The listing builds one solid part. Answer for the finished solid, in the listing's coordinates (mm). Face numbers are marked on the shaded views. A direction names the side the tool comes from. Round coordinates to 2 decimals unless told otherwise and drop trailing zeros. Order: outer loops, then holes, each group sorted by start corner. A loop starts at its lowest first (then second) coordinate and runs counter-clockwise, first axis right, second up. Notation, with made-up numbers: M -6.75,28 L 42.25,28 A32 ccw 42.25,58 Z; hole C 86.5,18 d8. An arc over 180 degrees is marked long. Put each result on its own line as item: value. Start each with the question number.
1. Each of these flat-tipped pins is pushed along its axis until it touches: pin 1 Ø8 at (y, z) = (-6.5, 25.5) entering from +X; pin 2 Ø1.5 at (x, z) = (20.5, 53.5) entering from -Y; pin 3 Ø6.5 at (x, y) = (-15, 10.5) entering from -Z; pin 4 Ø3 at (x, z) = (-17.5, -45) entering from -Y. Where does it stop, or does it pass through?
2. Which of the six approach directions +Z, -Z, +X, -X, +Y, -Y give full straight-line access (tool end or side, diameter ignored) to the marked faces 4, 5 and 6?
3. The mould has two halves that part along Z. Classify the marked faces 1, 2 and 3: +Z half, -Z half, draft (parallel to the pull), parting line (faces both ways), or undercut.
4. The part is cut by section B-B (x = 10). Give the vertices of the cut face in (y, z), then the cut area to 3 significant figures.
5. Consider line 1 (X direction, y = 1.5, z = -45); line 2 (X direction, y = 5.5, z = 9); line 3 (X direction, y = 10, z = 57). Determine where each line is inside the solid, lowest interval first.
6. The part is cut by section C-C (z = 32). Give the vertices of the cut face in (x, y).
7. The part is cut by section D-D (y = 10.5). Give the vertices of the cut face in (x, z), then the cut area to 3 significant figures.
8. The part is cut by section A-A (y = -3). Give the vertices of the cut face in (x, z), then the cut area to 3 significant figures.
from build123d import *

# Parameters (mm, degrees)
ESBO_O1_W                 = 90
ESBO_O1_H                 = 100
RESSALTO_EXTRUS_O1_DEPTH  = 3
ESBO_O4_W                 = 20
ESBO_O4_H                 = 20
CORTE_EXTRUS_O1_DEPTH     = 3
DOBRA_START               = -30
DOBRA_ESBO_ADA1_DEPTH     = 80
DOBRA_ESBO_ADA1_2_DEPTH   = 80
DOBRA_ESBO_ADA2_DEPTH     = 80
DOBRA_ESBO_ADA2_2_DEPTH   = 80
FILETE1_R                 = 5
CHANFRO1_SIZE             = 5
FILETE2_R                 = 2.5
ESBO_O7_R                 = 2.5
CORTE_EXTRUS_O2_DEPTH     = 3
RESSALTO_EXTRUS_O2_DEPTH  = 21.5
ESBO_O9_W                 = 37
ESBO_O9_H                 = 15
CORTE_EXTRUS_O7_DEPTH     = 90
ESBO_O10_W                = 3
ESBO_O10_H                = 20
RESSALTO_EXTRUS_O3_DEPTH  = 30
FURO_ROSCADO_DE_M51_D     = 4.2
FURO_ROSCADO_DE_M51_DEPTH = 14
FURO_ROSCADO_DE_M51_TIP   = 1.2618073


# Read off the part's stored shape, not the designer's step: Dobra esboçada1, Dobra esboçada2
with BuildPart() as part:
    # Esboço1 → Ressalto-extrusão1 (new body)
    with BuildSketch(Plane(origin=(0, 0, 0), x_dir=(1, 0, 0), z_dir=(0, 1, 0))):
        Rectangle(ESBO_O1_W, ESBO_O1_H)
    extrude(amount=RESSALTO_EXTRUS_O1_DEPTH)

    # Esboço4 → Corte-extrusão1 (cut)
    with BuildSketch(Plane(origin=(0, 3, 0), x_dir=(1, 0, 0), z_dir=(0, 1, 0))):
        with Locations((-35, 40)):
            Rectangle(ESBO_O4_W, ESBO_O4_H)
        with Locations((35, 40)):
            Rectangle(ESBO_O4_W, ESBO_O4_H)
    extrude(amount=-CORTE_EXTRUS_O1_DEPTH, mode=Mode.SUBTRACT)

    # Dobra esboçada1 outline → Dobra esboçada1 (cut)
    with BuildSketch(Plane.XY.offset(DOBRA_START)):
        with BuildLine():
            Line((-45, 0), (-28.872983346, 0))
            ThreePointArc((-28.872983346, 0), (-27.449489743, 2.16227766), (-25, 3))
            Line((-25, 3), (-45, 3))
            Line((-45, 3), (-45, 0))
        make_face()
    extrude(amount=DOBRA_ESBO_ADA1_DEPTH, mode=Mode.SUBTRACT)

    # Dobra esbo_ada1 2 outline → Dobra esbo_ada1 2 (add)
    with BuildSketch(Plane.XY.offset(DOBRA_START)):
        with BuildLine():
            ThreePointArc((-28.872983346, 0), (-28.968118785, -0.49598283), (-29, -1))
            Line((-29, -1), (-29, -17.073009183))
            Line((-29, -17.073009183), (-26, -17.073009183))
            Line((-26, -17.073009183), (-26, -1))
            ThreePointArc((-26, -1), (-25.707106781, -0.292893219), (-25, 0))
            Line((-25, 0), (-28.872983346, 0))
        make_face()
    extrude(amount=DOBRA_ESBO_ADA1_2_DEPTH)

    # Dobra esboçada2 outline → Dobra esboçada2 (cut)
    with BuildSketch(Plane.XY.offset(DOBRA_START)):
        with BuildLine():
            ThreePointArc((25, 3), (27.449489743, 2.16227766), (28.872983346, 0))
            Line((28.872983346, 0), (45, 0))
            Line((45, 0), (45, 3))
            Line((45, 3), (25, 3))
        make_face()
    extrude(amount=DOBRA_ESBO_ADA2_DEPTH, mode=Mode.SUBTRACT)

    # Dobra esbo_ada2 2 outline → Dobra esbo_ada2 2 (add)
    with BuildSketch(Plane.XY.offset(DOBRA_START)):
        with BuildLine():
            Line((26, -1), (26, -17.073009183))
            Line((26, -17.073009183), (29, -17.073009183))
            Line((29, -17.073009183), (29, -1))
            ThreePointArc((29, -1), (28.968118785, -0.49598283), (28.872983346, 0))
            Line((28.872983346, 0), (25, 0))
            ThreePointArc((25, 0), (25.707106781, -0.292893219), (26, -1))
        make_face()
    extrude(amount=DOBRA_ESBO_ADA2_2_DEPTH)

    # Filete1
    filete1_edges = [part.edges().sort_by_distance(p)[0] for p in [
        (-25, 1.5, -50),
        (25, 1.5, -50),
    ]]
    fillet(filete1_edges, radius=FILETE1_R)

    # Chanfro1
    chanfro1_edges = [part.edges().sort_by_distance(p)[0] for p in [
        (27.5, -17.073009183, -30),
        (27.5, -17.073009183, 50),
        (-27.5, -17.073009183, -30),
        (-27.5, -17.073009183, 50),
    ]]
    chamfer(chanfro1_edges, length=CHANFRO1_SIZE)

    # Filete2
    filete2_edges = [part.edges().sort_by_distance(p)[0] for p in [
        (27.5, -12.073009183, 50),
        (27.5, -17.073009183, -25),
        (27.5, -17.073009183, 45),
        (-27.5, -17.073009183, -25),
        (-27.5, -17.073009183, 45),
        (-27.5, -12.073009183, 50),
        (27.5, -12.073009183, -30),
        (-27.5, -12.073009183, -30),
    ]]
    fillet(filete2_edges, radius=FILETE2_R)

    # Esboço7 → Corte-extrusão2 (cut)
    with BuildSketch(Plane(origin=(0, 3, 0), x_dir=(1, 0, 0), z_dir=(0, 1, 0))):
        with Locations(Location((-17.5, 45, 0), (0, 0, 270))):
            Circle(ESBO_O7_R)
        with Locations(Location((17.5, 45, 0), (0, 0, 270))):
            Circle(ESBO_O7_R)
    extrude(amount=-CORTE_EXTRUS_O2_DEPTH, mode=Mode.SUBTRACT)

    # Esboço8 → Ressalto-extrusão2 (add, symmetric)
    with BuildSketch(Plane(origin=(0, 0, 0), x_dir=(0, 0, -1), z_dir=(1, 0, 0))):
        Polygon((30, 3), (-25.980762114, 18), (-55.980762114, 18), (-55.980762114, 3), align=None)
    extrude(amount=RESSALTO_EXTRUS_O2_DEPTH, both=True)

    # Esboço9 → Corte-extrusão7 (cut)
    with BuildSketch(Plane.XY.offset(55.980762114)):
        with Locations((0, 10.5)):
            Rectangle(ESBO_O9_W, ESBO_O9_H)
    extrude(amount=-CORTE_EXTRUS_O7_DEPTH, mode=Mode.SUBTRACT)

    # Esboço10 → Ressalto-extrusão3 (add, symmetric)
    with BuildSketch(Plane(origin=(0, 0, 0), x_dir=(0, 0, -1), z_dir=(1, 0, 0))):
        with Locations((-57.480762114, 10.5)):
            Rectangle(ESBO_O10_W, ESBO_O10_H)
    extrude(amount=RESSALTO_EXTRUS_O3_DEPTH, both=True)

    # Furo roscado de M51
    with Locations(Plane.XY.offset(58.980762114)):
        with Locations((-15, 10.5), (15, 10.5)):
            Hole(FURO_ROSCADO_DE_M51_D / 2, depth=FURO_ROSCADO_DE_M51_DEPTH)
            with Locations((0, 0, -(FURO_ROSCADO_DE_M51_DEPTH + FURO_ROSCADO_DE_M51_TIP / 2))):  # 118° drill point
                Cone(0, FURO_ROSCADO_DE_M51_D / 2, FURO_ROSCADO_DE_M51_TIP, mode=Mode.SUBTRACT)


solid = part.part
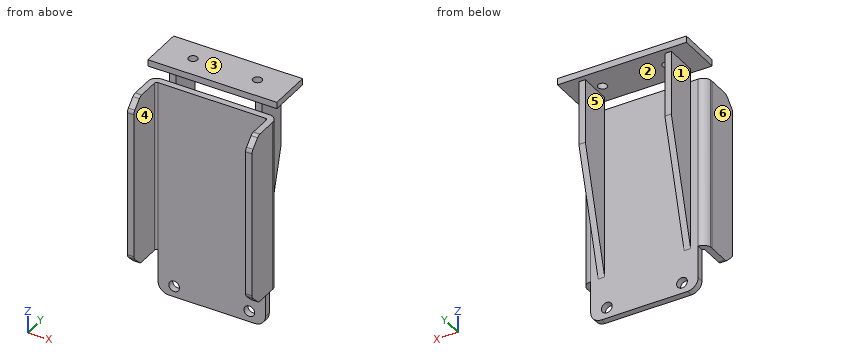
Resolved:
1. pin 1: x = 29
1. pin 2: y = 3
1. pin 3: z = 55.98
1. pin 4: through
2. face 4: +Z, -Z, -Y
2. face 5: -Z, +Y
2. face 6: +Z, -Z, -X, +Y, -Y
3. face 1: draft
3. face 2: undercut
3. face 3: +Z half
4. outline: M 0,-50 L 3,-50 L 3,50 L 0,50 Z; M 0.5,55.98 L 20.5,55.98 L 20.5,58.98 L 0.5,58.98 Z
4. area: 360 mm2
5. line 1: -25 to -20, -15 to 15, 20 to 25
5. line 2: -21.5 to -18.5, 18.5 to 21.5
5. line 3: -30 to -17.04, -12.96 to 12.96, 17.04 to 30
6. outline: M -29,-17.07 L -26,-17.07 L -26,-1 A1 cw -25,0 L 25,0 A1 cw 26,-1 L 26,-17.07 L 29,-17.07 L 29,-1 A4 ccw 25,3 L 21.5,3 L 21.5,18 L 18.5,18 L 18.5,3 L -18.5,3 L -18.5,18 L -21.5,18 L -21.5,3 L -25,3 A4 ccw -29,-1 Z
7. outline: M -30,55.98 L -21.5,55.98 L -21.5,-2.01 L -18.5,-2.01 L -18.5,55.98 L -17.1,55.98 L -17.1,58.98 L -30,58.98 Z; M -12.9,55.98 L 12.9,55.98 L 12.9,58.98 L -12.9,58.98 Z; M 17.1,55.98 L 18.5,55.98 L 18.5,-2.01 L 21.5,-2.01 L 21.5,55.98 L 30,55.98 L 30,58.98 L 17.1,58.98 Z
7. area: 503 mm2
8. outline: M -29,-30 L -26,-30 L -26,50 L -29,50 Z; M 26,-30 L 29,-30 L 29,50 L 26,50 Z
8. area: 480 mm2
